from build123d import *

# Parameters (mm, degrees)
F0_R     = 54.205812
F0_R_2   = 41.292584
F1_DEPTH = 205
F4_R     = 41.024739
F4_R_2   = 33.495835
F5_DEPTH = 342.6


with BuildPart() as f1:
    # F0 (on Front) → F1 (new body)
    with BuildSketch(Plane.XZ):
        Circle(F0_R)
        Circle(F0_R_2, mode=Mode.SUBTRACT)
    extrude(amount=F1_DEPTH)

    # F2 (on Right) → F3 (revolve)
    with BuildSketch(Plane.YZ):
        Polygon((0, 54.346781), (0, 0), (74.203447, 0), align=None)
    revolve(axis=Axis((0, 37.101723, 0), (0, 1, 0)))

    # F4 (on Front) → F5 (join)
    with BuildSketch(Plane.XZ):
        Circle(F4_R)
        Circle(F4_R_2, mode=Mode.SUBTRACT)
    extrude(amount=F5_DEPTH)


solid = f1.part
Geometry: final body of the model. Coordinates: model frame, mm. A direction names the side the tool comes from. Give positions to 0.01 mm unless a question says otherwise; leave off trailing zeros. Write each loop counter-clockwise with the first axis right and the second up, starting at its lowest first coordinate (ties: lowest second). Pieces come first, ordered by that corner, then holes.
(1) Cut plane A-A, the plane y = -127. Return loops of the section in (x, z).
(2) Mould query, pull axis Z, two halves, no side actions, for faces 3 (the cylindrical face through (-8.89, -168.9, -40.05)), 4 (the cylindrical face through (29.141, -101.065, 45.707)), 5 (the flat face through (-12, -205, -40)). Classes: released by +Z, released by -Z, zero draft, split by the parting line, or undercut.
(3) First-contact query: P1, Ø8, axis at x = 9.5, y = -134, coming from the -Z side; P2, Ø10, axis at y = -130.5, z = -25, coming from the -X side; P3, Ø12, axis at y = -64.5, z = -14, coming from the +X side. Flat tips, straight axial feed; report the tip coordinate or a pass-through.
(4) Ray query, line 1 (X direction, y = -143.5, z = 2); line 2 (Z direction, x = 0, y = -149); line 3 (Z direction, x = 8.5, y = -136.5). Return the intervals inside material, ascending.
(5) Access query for faces 1 (the cylindrical face through (-9, -101.1, -40.3)), 2 (the conical face through (-15.11, 53.07, -3.36)). Directions: +Z, -Z, +X, -X, +Y, -Y. A direction counts if a zero-diameter tool reaches every point of the face in a straight line with its end or side. Return the directions, or none.
Values follow:
1. outline: circle Ø108.41 at (0, 0); circle Ø82.05 at (0, 0); hole circle Ø82.59 at (0, 0); hole circle Ø66.99 at (0, 0)
2. face 3: undercut
2. face 4: split by the parting line
2. face 5: zero draft
3. P1: stops at z = -53.93
3. P2: stops at x = -50.38
3. P3: stops at x = 53.61
4. line 1: x = -54.17 to -41.24, -40.98 to -33.44, 33.44 to 40.98, 41.24 to 54.17
4. line 2: z = -54.21 to -41.29, -41.02 to -33.5, 33.5 to 41.02, 41.29 to 54.21
4. line 3: z = -53.54 to -40.41, -40.13 to -32.4, 32.4 to 40.13, 40.41 to 53.54
5. face 1: -Y
5. face 2: +Y
